Part model, mm, in its own coordinate system. Face numbers are marked on the shaded views. Give positions to 0.01 mm unless a question says otherwise; leave off trailing zeros. Write each loop counter-clockwise with the first axis right and the second up, starting at its lowest first coordinate (ties: lowest second). Pieces come first, ordered by that corner, then holes.
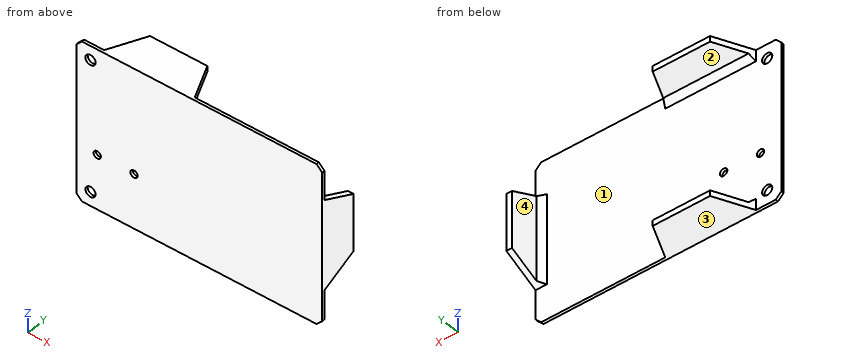
```python
from build123d import *

# Parameters (mm, degrees)
SKETCH1_W           = 110.236
SKETCH1_H           = 72.136
BOSS_EXTRUDE1_DEPTH = 1.27
SKETCH2_R           = 2.286
SKETCH2_R_2         = 1.651
CUT_EXTRUDE1_DEPTH  = 1.27
SKETCH3_W           = 25.4
SKETCH3_H           = 2.54
SKETCH3_W_2         = 2.54
SKETCH3_H_2         = 25.4
BOSS_EXTRUDE2_DEPTH = 16
CHAMFER1_SIZE       = 7.62
CHAMFER1_SIZE_2     = 16.341142734
CHAMFER2_SIZE       = 2.54
CHAMFER3_SIZE       = 2.54


with BuildPart() as part:
    # Sketch1 → Boss-Extrude1 (new body)
    with BuildSketch(Plane(origin=(0, 0, 0), x_dir=(1, 0, 0), z_dir=(0, 1, 0))):
        with Locations((55.118, 36.068)):
            Rectangle(SKETCH1_W, SKETCH1_H)
    extrude(amount=BOSS_EXTRUDE1_DEPTH)

    # Sketch2 → Cut-Extrude1 (cut)
    with BuildSketch(Plane(origin=(0, 1.27, 0), x_dir=(1, 0, 0), z_dir=(0, 1, 0))):
        with Locations(Location((6.35, 65.786, 0), (0, 0, 270))):
            Circle(SKETCH2_R)
        with Locations(Location((9.363, 47.498, 0), (0, 0, 270))):
            Circle(SKETCH2_R_2)
        with Locations(Location((25.873, 47.498, 0), (0, 0, 270))):
            Circle(SKETCH2_R_2)
        with Locations(Location((6.35, 6.35, 0), (0, 0, 90))):
            Circle(SKETCH2_R)
    extrude(amount=-CUT_EXTRUDE1_DEPTH, mode=Mode.SUBTRACT)

    # Sketch3 → Boss-Extrude2 (add)
    with BuildSketch(Plane(origin=(0, 1.27, 0), x_dir=(1, 0, 0), z_dir=(0, 1, 0))):
        with Locations((31.75, 70.866)):
            Rectangle(SKETCH3_W, SKETCH3_H)
        with Locations((31.75, 1.27)):
            Rectangle(SKETCH3_W, SKETCH3_H)
        with Locations((108.966, 36.068)):
            Rectangle(SKETCH3_W_2, SKETCH3_H_2)
    extrude(amount=BOSS_EXTRUDE2_DEPTH)

    # Chamfer1
    # the kernel refuses this chamfer: 16.341142734, 7.62 mm, written as the material it adds along each edge
    with BuildSketch(Plane(origin=(44.45, 1.27, -2.54), x_dir=(0.9971975577536774, -0.07481330637060034, 0), z_dir=(0, 0, 1))) as chamfer1_piece_1_section:
        Polygon((CHAMFER1_SIZE * 0.997197557754, CHAMFER1_SIZE * 0.0748133063706), (-CHAMFER1_SIZE_2 * 0.0748133063719, CHAMFER1_SIZE_2 * 0.997197557771), (0, 0), align=None)
    chamfer1_piece_1 = extrude(amount=2.54, mode=Mode.PRIVATE)
    chamfer1_piece_1 = split(chamfer1_piece_1, bisect_by=Plane(origin=(46.87141812, 17.27, -1.27), z_dir=(0, -1, 0)), keep=Keep.TOP, mode=Mode.PRIVATE)
    add(chamfer1_piece_1)
    with BuildSketch(Plane(origin=(44.45, 1.27, -72.136), x_dir=(0.9971975577536774, -0.07481330637060034, 2.7895727589747506e-15), z_dir=(0, 0, 1))) as chamfer1_piece_2_section:
        Polygon((CHAMFER1_SIZE * 0.997197557754, CHAMFER1_SIZE * 0.0748133063706), (-CHAMFER1_SIZE_2 * 0.0748133063719, CHAMFER1_SIZE_2 * 0.997197557771), (0, 0), align=None)
    chamfer1_piece_2 = extrude(amount=2.54, mode=Mode.PRIVATE)
    chamfer1_piece_2 = split(chamfer1_piece_2, bisect_by=Plane(origin=(46.87141812, 17.27, -70.866), z_dir=(0, -1, 0)), keep=Keep.TOP, mode=Mode.PRIVATE)
    add(chamfer1_piece_2)
    with BuildSketch(Plane(origin=(19.05, 1.27, 0), x_dir=(-0.9971975577536774, -0.07481330637060028, 0), z_dir=(0, 0, -1))) as chamfer1_piece_3_section:
        Polygon((CHAMFER1_SIZE * 0.997197557754, CHAMFER1_SIZE * 0.0748133063706), (-CHAMFER1_SIZE_2 * 0.0748133063719, CHAMFER1_SIZE_2 * 0.997197557771), (0, 0), align=None)
    chamfer1_piece_3 = extrude(amount=2.54, mode=Mode.PRIVATE)
    chamfer1_piece_3 = split(chamfer1_piece_3, bisect_by=Plane(origin=(16.62858188, 17.27, -1.27), z_dir=(0, -1, 0)), keep=Keep.TOP, mode=Mode.PRIVATE)
    add(chamfer1_piece_3)
    with BuildSketch(Plane(origin=(19.05, 1.27, -69.596), x_dir=(-0.9971975577536774, -0.07481330637060032, 5.5791455179495004e-15), z_dir=(0, 0, -1))) as chamfer1_piece_4_section:
        Polygon((CHAMFER1_SIZE * 0.997197557754, CHAMFER1_SIZE * 0.0748133063706), (-CHAMFER1_SIZE_2 * 0.0748133063719, CHAMFER1_SIZE_2 * 0.997197557771), (0, 0), align=None)
    chamfer1_piece_4 = extrude(amount=2.54, mode=Mode.PRIVATE)
    chamfer1_piece_4 = split(chamfer1_piece_4, bisect_by=Plane(origin=(16.62858188, 17.27, -70.866), z_dir=(0, -1, 0)), keep=Keep.TOP, mode=Mode.PRIVATE)
    add(chamfer1_piece_4)
    with BuildSketch(Plane(origin=(107.696, 1.27, -48.768), x_dir=(0, -0.07481330637060034, -0.9971975577536774), z_dir=(1, 0, 0))) as chamfer1_piece_5_section:
        Polygon((CHAMFER1_SIZE * 0.997197557754, CHAMFER1_SIZE * 0.0748133063706), (-CHAMFER1_SIZE_2 * 0.0748133063719, CHAMFER1_SIZE_2 * 0.997197557771), (0, 0), align=None)
    chamfer1_piece_5 = extrude(amount=2.54, mode=Mode.PRIVATE)
    chamfer1_piece_5 = split(chamfer1_piece_5, bisect_by=Plane(origin=(108.966, 17.27, -51.18941812), z_dir=(0, -1, 0)), keep=Keep.TOP, mode=Mode.PRIVATE)
    add(chamfer1_piece_5)
    with BuildSketch(Plane(origin=(110.236, 1.27, -23.368), x_dir=(0, -0.07481330637060032, 0.9971975577536774), z_dir=(-1, 0, 0))) as chamfer1_piece_6_section:
        Polygon((CHAMFER1_SIZE * 0.997197557754, CHAMFER1_SIZE * 0.0748133063706), (-CHAMFER1_SIZE_2 * 0.0748133063719, CHAMFER1_SIZE_2 * 0.997197557771), (0, 0), align=None)
    chamfer1_piece_6 = extrude(amount=2.54, mode=Mode.PRIVATE)
    chamfer1_piece_6 = split(chamfer1_piece_6, bisect_by=Plane(origin=(108.966, 17.27, -20.94658188), z_dir=(0, -1, 0)), keep=Keep.TOP, mode=Mode.PRIVATE)
    add(chamfer1_piece_6)

    # Chamfer2
    chamfer2_edges = [part.edges().sort_by_distance(p)[0] for p in [
        (31.75, 1.27, -69.596),
        (31.75, 1.27, -2.54),
        (107.696, 1.27, -36.068),
    ]]
    chamfer(chamfer2_edges, length=CHAMFER2_SIZE)

    # Chamfer3
    chamfer3_edges = [part.edges().sort_by_distance(p)[0] for p in [
        (0, 0.635, -72.136),
        (110.236, 0.635, -72.136),
        (110.236, 0.635, 0),
        (0, 0.635, 0),
    ]]
    chamfer(chamfer3_edges, length=CHAMFER3_SIZE)


solid = part.part
```
1) Saw through at B-B, the plane z = -6.35. Write the cut outline in (x, y).
Answers follow:
outline: (0, 0) - (4.06, 0) - (4.06, 1.27) - (0, 1.27) - close; (8.64, 0) - (110.24, 0) - (110.24, 1.27) - (8.64, 1.27) - close
2) Saw through at D-D, the plane z = -31.5. Write the cut outline in (x, y).
Answers follow:
outline: (0, 0) - (110.24, 0) - (110.24, 17.27) - (107.7, 17.27) - (107.7, 3.81) - (105.16, 1.27) - (0, 1.27) - close
3) Two-plate mould, pull along Z, no slides. Class the marked faces 1, 2, 3 and 4: +Z half, -Z half, draft (parallel to the pull), parting line (faces both ways), or undercut.
Answers follow:
face 1: undercut
face 2: undercut
face 3: -Z half
face 4: draft
4) Saw through at C-C, the plane y = 11.5. Write the cut outline in (x, z), then the cut area to 3 significant figures.
Answers follow:
outline: (16.2, -72.14) - (47.3, -72.14) - (47.3, -69.6) - (16.2, -69.6) - close; (16.2, -2.54) - (47.3, -2.54) - (47.3, 0) - (16.2, 0) - close; (107.7, -51.62) - (110.24, -51.62) - (110.24, -20.52) - (107.7, -20.52) - close
area: 237 mm2
5) Saw through at A-A, the plane x = 6.35. Write the cut outline in (y, z), then the cut area to 3 significant figures.
Answers follow:
outline: (0, -72.14) - (1.27, -72.14) - (1.27, -68.07) - (0, -68.07) - close; (0, -63.5) - (1.27, -63.5) - (1.27, -8.64) - (0, -8.64) - close; (0, -4.06) - (1.27, -4.06) - (1.27, 0) - (0, 0) - close
area: 80.0 mm2
6) Wall check: L1, parallel to Z at x = 26.5, y = 5; L2, parallel to X at y = 0.9, z = -6.35; L3, parallel to Y at x = 8.5, z = -53.5. Give the ranges that are in metal, low to high.
Answers follow:
L1: z = -72.14 to -69.6, -2.54 to 0
L2: x = 0 to 4.06, 8.64 to 110.24
L3: y = 0 to 1.27
7) Pin check, flat tips, straight feed: pin 1 Ø6 at (x, z) = (21.5, -23) entering from +Y; pin 2 Ø2.5 at (x, z) = (9.363, -47.498) entering from -Y; pin 3 Ø4 at (y, z) = (12, -42) entering from -X. Stop position of each tip, or through.
Answers follow:
pin 1: stops at y = 1.27
pin 2: passes through
pin 3: stops at x = 107.7
